```python
from build123d import *

# Parameters (mm, degrees)
EXTRUDE_2_DEPTH = 5
SKETCH_5_W      = 20
SKETCH_5_H      = 20
SKETCH_5_R      = 4
EXTRUDE_3_DEPTH = 15
FILLET_1_R      = 8


with BuildPart() as part:
    # 草图3 → 凸台-拉伸2 (new, symmetric)
    with BuildSketch(Plane(origin=(0, 0, 0), x_dir=(0, 0, -1), z_dir=(1, 0, 0))):
        Polygon((31, 0), (46, 0), (46, 100), (-46, 100), (-46, 0), (-31, 0), (-31, 90), (31, 90), align=None)
    extrude(amount=EXTRUDE_2_DEPTH, both=True)

    # 草图5 → 凸台-拉伸3 (add)
    with BuildSketch(Plane.XY.offset(46)):
        with Locations((-5, 110)):
            Rectangle(SKETCH_5_W, SKETCH_5_H)
        with Locations((-5, 110)):
            Circle(SKETCH_5_R, mode=Mode.SUBTRACT)
    extrude_3 = extrude(amount=-EXTRUDE_3_DEPTH)

    # 镜向1: 凸台-拉伸3 across plane
    add(extrude_3.mirror(Plane.XY))

    # 圆角1
    fillet_1_edges = [part.edges().sort_by_distance(p)[0] for p in [
        (-5, 100, -38.5),
        (-5, 100, 38.5),
    ]]
    fillet(fillet_1_edges, radius=FILLET_1_R)


solid = part.part
```
The listing builds one solid part. Answer for the finished solid, in the listing's coordinates (mm). A direction names the side the tool comes from. Give positions to 0.01 mm unless a question says otherwise; leave off trailing zeros. Loops run counter-clockwise (first coordinate to the right, second up) from the corner with the lowest first, then second, coordinate; pieces in that order, holes last. Notation, with made-up numbers: (5, 13.5) - (9, 13.5) arc R18 cw to (9, 24.5) - close; hole circle Ø8 at (-21, 61). An arc over 180 degrees is marked (long way). Answer as CSV lines item,"result". Start each with the question number.
Item 1: Each of these flat-tipped pins is pushed along its axis until it touches: pin 1 (7 mm diameter, centred on x = -5, y = 110, fed in from -Z); pin 2 (2 mm diameter, centred on x = -14, z = 36, fed in from -Y); pin 3 (12 mm diameter, centred on x = -7.5, z = -6.5, fed in from +Y); pin 4 (12 mm diameter, centred on y = 34.5, z = 31.5, fed in from -X). Where does it stop, or does it pass through?
Item 2: The mould has two halves that part along Y. Classify faces 1 (the face through (-5, 50.7, 31.3)), 2 (the face through (-5.521, 113.966, -38.605)), 3 (the face through (-5, 120, -39)): +Y half, -Y half, draft (parallel to the pull), parting line (faces both ways), or undercut.
Item 3: A cutting plane is placed at C-C on x = 3. Determine the outline of the cut face in (y, z).
Item 4: A cutting plane is placed at D-D on y = 110. Determine the outline of the cut face in (x, z).
Item 5: A cutting plane is placed at A-A on y = 80. Determine the outline of the cut face in (x, z), then the cut area to 3 significant figures.
Item 6: A cutting plane is placed at B-B on z = 36. Determine the outline of the cut face in (x, y), then the cut area to 3 significant figures.
Item 7: For faces 4 (the face through (0, 90, 0)), 5 (the face through (0, 100, 0)), 6 (the face through (5, 72.5, -31.3)), determine the directions among +Z, -Z, +X, -X, +Y, -Y from which every point of the face is accessible in a straight line to the end or side of a thin tool.
Item 8: Find the intervals of material crossed by line 1 (Z direction, x = -1.75, y = 87.5); line 2 (Y direction, x = 1.25, z = -1.5); line 3 (X direction, y = 45, z = -42), in increasing order. Write a range as from..to.
Found:
1,pin 1,"passes through"
1,pin 2,"stops at y = 100"
1,pin 3,"stops at y = 100"
1,pin 4,"stops at x = -5"
2,face 1,"draft"
2,face 2,"undercut"
2,face 3,"+Y half"
3,outline,"(0, -46) - (120, -46) - (120, -31) - (100, -31) - (100, 31) - (120, 31) - (120, 46) - (0, 46) - (0, 31) - (90, 31) - (90, -31) - (0, -31) - close"
4,outline,"(-15, -46) - (-9, -46) - (-9, -31) - (-15, -31) - close; (-15, 31) - (-9, 31) - (-9, 46) - (-15, 46) - close; (-1, -46) - (5, -46) - (5, -31) - (-1, -31) - close; (-1, 31) - (5, 31) - (5, 46) - (-1, 46) - close"
5,outline,"(-5, -46) - (5, -46) - (5, -31) - (-5, -31) - close; (-5, 31) - (5, 31) - (5, 46) - (-5, 46) - close"
5,area,"300 mm^2"
6,outline,"(-15, 100) - (-13, 100) arc R8 cw to (-5, 92) - (-5, 0) - (5, 0) - (5, 120) - (-15, 120) - close; hole circle Ø8 at (-5, 110)"
6,area,"1,360 mm^2"
7,face 4,"+X, -X, -Y"
7,face 5,"+X, -X, +Y"
7,face 6,"+Z, -Z, +X, +Y, -Y"
8,line 1,"z = -46..-31, 31..46"
8,line 2,"y = 90..100"
8,line 3,"x = -5..5"
